from build123d import *

# Parameters (mm, degrees)
SKETCH1_R           = 46.2
BOSS_EXTRUDE1_DEPTH = 224
SHELL1_T            = -4
FILLET1_R           = 2
FILLET2_R           = 2
FILLET3_R           = 1
CHAMFER1_SIZE       = 1


with BuildPart() as part:
    # Sketch1 → Boss-Extrude1 (new body)
    with BuildSketch(Plane(origin=(0, 0, 0), x_dir=(1, 0, 0), z_dir=(0, 1, 0))):
        with Locations(Location((0, 0, 0), (0, 0, 270))):
            Circle(SKETCH1_R)
    extrude(amount=BOSS_EXTRUDE1_DEPTH)

    # Shell1
    shell1_openings = [part.faces().sort_by_distance(p)[0] for p in [
        (0, 224, 0),
    ]]
    offset(amount=SHELL1_T, openings=shell1_openings, kind=Kind.INTERSECTION)

    # Fillet1
    fillet1_edges = [part.edges().sort_by_distance(p)[0] for p in [
        (0, 4, -42.2),
    ]]
    fillet(fillet1_edges, radius=FILLET1_R)

    # Fillet2
    fillet2_edges = [part.edges().sort_by_distance(p)[0] for p in [
        (0, 224, -46.2),
    ]]
    fillet(fillet2_edges, radius=FILLET2_R)

    # Fillet3
    fillet3_edges = [part.edges().sort_by_distance(p)[0] for p in [
        (0, 224, -42.2),
    ]]
    fillet(fillet3_edges, radius=FILLET3_R)

    # Chamfer1
    chamfer1_edges = [part.edges().sort_by_distance(p)[0] for p in [
        (0, 0, -46.2),
    ]]
    chamfer(chamfer1_edges, length=CHAMFER1_SIZE)


solid = part.part
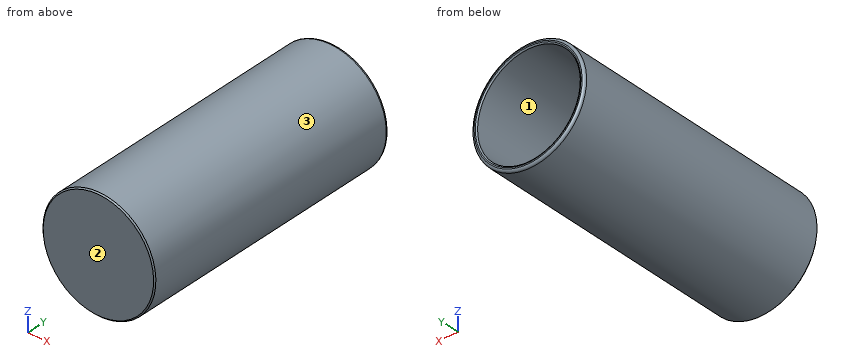
Can you work these out from the model? Positions are in its coordinate system, mm. Face numbers are marked on the shaded views. Give positions to 0.01 mm unless a question says otherwise; leave off trailing zeros. Loops run counter-clockwise (first coordinate to the right, second up) from the corner with the lowest first, then second, coordinate; pieces in that order, holes last. Notation, with made-up numbers: M 89,85 L 101,85 A30 ccw 101,123 Z; hole C 21.25,-7 d1. An arc over 180 degrees is marked long. One line per item, written item: value. Start each with the question number.
1) Thinking about a two-plate mould opening in Z: for the marked faces 1, 2 and 3, which applies, +Z half, -Z half, draft (parallel to the pull), parting line (faces both ways), or undercut?
2) If I drill on line 1 (X direction, y = 120, z = 0); line 2 (Y direction, x = 4, z = -39.5); line 3 (X direction, y = 53.5, z = -34.5), over which ranges is the centre line in solid material (lowest first)? Write a range as [from, to].
3) If we section it at B-B, the plane y = 125: Write out the boundary of the cut face in (x, z), and give its area (3 significant figures).
4) If we section it at C-C, the plane z = 0: Write out the boundary of the cut face in (x, y).
5) If we section it at A-A, the plane x = 0: Write out the boundary of the cut face in (y, z).
6) I'm going to push flat-ended pins straight in: pin 1 (8 mm diameter, centred on x = 30, y = 49.5, fed in from -Z); pin 2 (3 mm diameter, centred on x = 21.5, y = 131, fed in from +Z); pin 3 (5 mm diameter, centred on x = -20, z = 6, fed in from +Y). Where does each tip first touch, or does it pass through?
Completed:
1. face 1: undercut
1. face 2: draft
1. face 3: parting line
2. line 1: x = [-46.2, -42.2], [42.2, 46.2]
2. line 2: y = [0, 4]
2. line 3: x = [-30.73, -24.3], [24.3, 30.73]
3. outline: C 0,0 d92.4; hole C 0,0 d84.4
3. area: 1,110 mm^2
4. outline: M -46.2,1 L -45.2,0 L 45.2,0 L 46.2,1 L 46.2,222 A2 ccw 44.2,224 L 43.2,224 A1 ccw 42.2,223 L 42.2,6 A2 cw 40.2,4 L -40.2,4 A2 cw -42.2,6 L -42.2,223 A1 ccw -43.2,224 L -44.2,224 A2 ccw -46.2,222 Z
5. outline: M 0,-45.2 L 1,-46.2 L 222,-46.2 A2 ccw 224,-44.2 L 224,-43.2 A1 ccw 223,-42.2 L 6,-42.2 A2 cw 4,-40.2 L 4,40.2 A2 cw 6,42.2 L 223,42.2 A1 ccw 224,43.2 L 224,44.2 A2 ccw 222,46.2 L 1,46.2 L 0,45.2 Z
6. pin 1: stops at z = -38.19
6. pin 2: stops at z = 41.65
6. pin 3: stops at y = 4
